Study the drawing (mm; zero at the part's minimum x, y, z) and answer. A direction names the side the tool comes from. Round coordinates to 2 decimals unless told otherwise and drop trailing zeros. Order: outer loops, then holes, each group sorted by start corner. A loop starts at its lowest first (then second) coordinate and runs counter-clockwise, first axis right, second up. Notation, with made-up numbers: (16, -35) - (40, -35) arc R10 cw to (40, -18) - close; hole circle Ø9 at (0.5, -35). An arc over 180 degrees is marked (long way). Put each result on its own line as item: value.
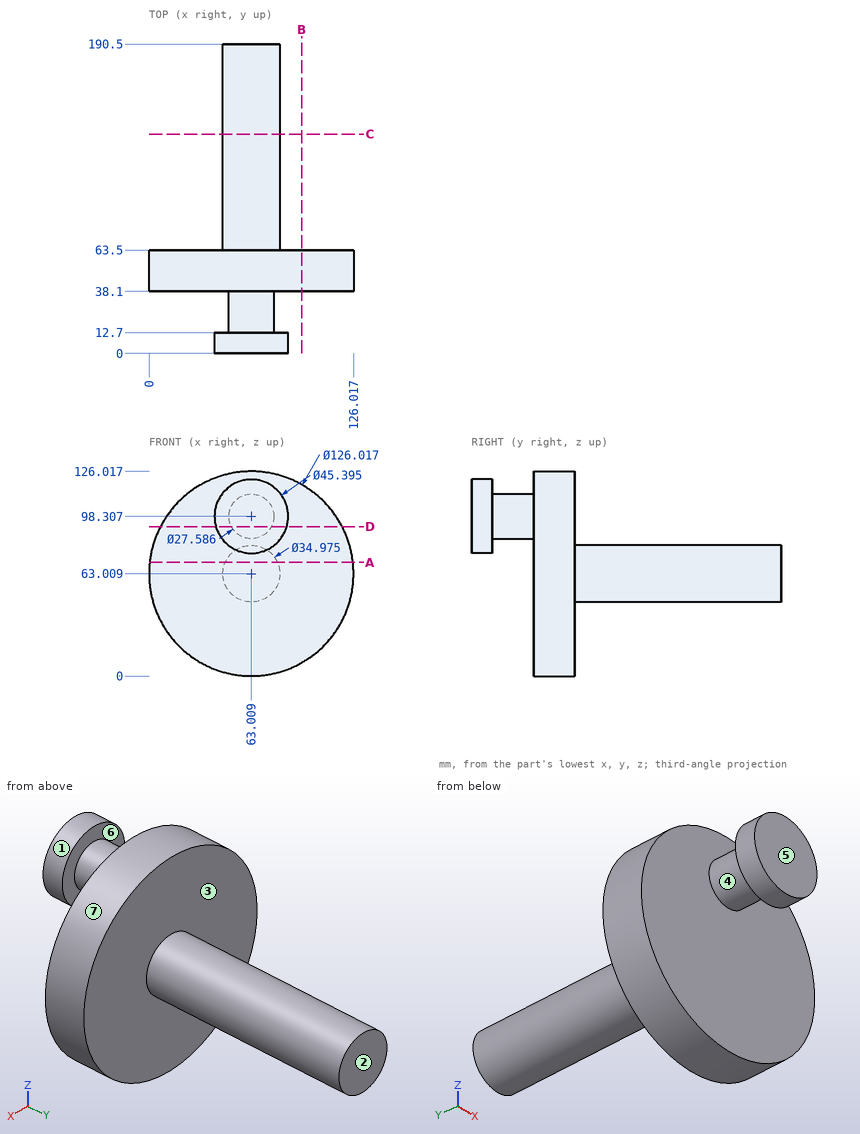
1) A cutting plane is placed at A-A on z = 70. Write down the section's boundary in (x, y), then the cut area to 3 significant figures.
Findings below:
outline: (0.39, 38.1) - (125.63, 38.1) - (125.63, 63.5) - (79.04, 63.5) - (79.04, 190.5) - (46.98, 190.5) - (46.98, 63.5) - (0.39, 63.5) - close
area: 7,250 mm2
2) For a pull along Y with two mould halves and no side action, classify the marked faces 4, 5, 6 and 7 as pulls with the +Y half, pulls with the -Y half, needs draft (parallel to the pull), parting line crosses it, or undercut.
Findings below:
face 4: undercut
face 5: pulls with the -Y half
face 6: undercut
face 7: needs draft
3) For the marked faces 1, 2 and 3, determine the directions among +Z, -Z, +X, -X, +Y, -Y from which every point of the face is accessible in a straight line to the end or side of a thin tool.
Findings below:
face 1: -Y
face 2: +Z, -Z, +X, -X, +Y
face 3: +Y
4) A cutting plane is placed at B-B on x = 94. Write down the section's boundary in (y, z), then the cut area to 3 significant figures.
Findings below:
outline: (38.1, 8.15) - (63.5, 8.15) - (63.5, 117.87) - (38.1, 117.87) - close
area: 2,790 mm2
5) Given pin 1 Ø8 at (x, z) = (99, 30.5) entering from -Y; pin 2 Ø8 at (y, z) = (43.5, 97) entering from +X; pin 3 Ø1 at (x, z) = (17, 93) entering from +Y, each flat-ended and moving along its own axis, determine where each tip first touches the part or whether it passes through.
Findings below:
pin 1: stops at y = 38.1
pin 2: stops at x = 118.42
pin 3: stops at y = 63.5
6) A cutting plane is placed at D-D on z = 92. Write down the section's boundary in (x, y) (1 decimal).
Findings below:
outline: (7.1, 38.1) - (50.7, 38.1) - (50.7, 12.7) - (41.2, 12.7) - (41.2, 0) - (84.8, 0) - (84.8, 12.7) - (75.3, 12.7) - (75.3, 38.1) - (119, 38.1) - (119, 63.5) - (7.1, 63.5) - close
7) Straight lines are drawn through the part: L1, parallel to Y at x = 47.5, z = 106; L2, parallel to Y at x = 116, z = 95.5; L3, parallel to Y at x = 60.5, z = 88. For each, find the intervals that lie inside material, in ascending order. Write a range as from..to.
Findings below:
L1: y = 0..12.7, 38.1..63.5
L2: y = 38.1..63.5
L3: y = 0..63.5
8) A cutting plane is placed at C-C on y = 135. Write down the section's boundary in (x, z) (1 decimal), then the cut area to 3 significant figures.
Findings below:
outline: circle Ø35 at (63, 63)
area: 961 mm2
